Here's how the part is built. I have some questions about the finished solid (model axes, mm). Round coordinates to 2 decimals unless told otherwise and drop trailing zeros. Write each loop counter-clockwise with the first axis right and the second up, starting at its lowest first coordinate (ties: lowest second). Pieces come first, ordered by that corner, then holes. Notation, with made-up numbers: (21.25, -7) - (77.25, -7) arc R33 ccw to (77.25, 31) - close; hole circle Ø5 at (-37.75, 34). An arc over 180 degrees is marked (long way). Return JSON: item names as keys, results as strings. Group by question number.
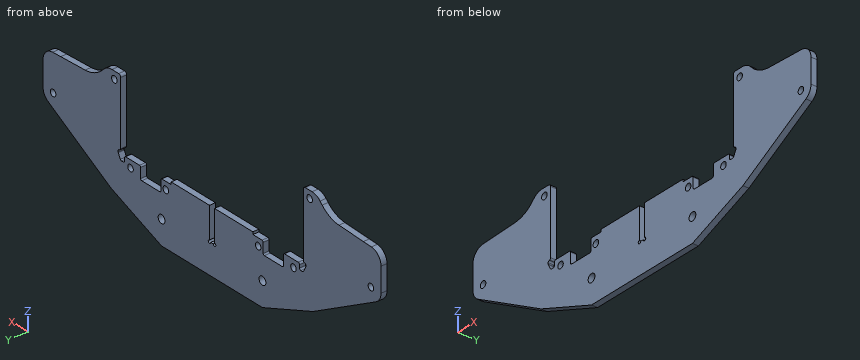
```python
from build123d import *

# Parameters (mm, degrees)
EXTRUDE_1_DEPTH      = 2
CUT_EXTRUDE_1_DEPTH  = 10
SKETCH_3_W           = 2
SKETCH_3_H           = 10
CUT_EXTRUDE_2_DEPTH  = 10
CUT_EXTRUDE_3_DEPTH  = 10
SKETCH_5_W           = 23
SKETCH_5_H           = 22.484633815
CUT_EXTRUDE_4_DEPTH  = 10
SKETCH_6_W           = 32.4
SKETCH_6_H           = 0.8
EXTRUDE_2_DEPTH      = 2
SKETCH_7_R           = 1.1
CUT_EXTRUDE_5_DEPTH  = 10
EXTRUDE_3_DEPTH      = 2
SKETCH_9_R           = 1.1
CUT_EXTRUDE_6_DEPTH  = 10
CHAMFER_2_SIZE       = 5
CHAMFER_2_SIZE_2     = 5.237723549
FILLET_2_R           = 10
FILLET_3_R           = 4.5
SKETCH_10_W          = 1.5
SKETCH_10_H          = 2
CUT_EXTRUDE_7_DEPTH  = 10
SKETCH_11_R          = 1.35
CUT_EXTRUDE_8_DEPTH  = 10
SKETCH_12_W          = 8
SKETCH_12_H          = 4.2
CUT_EXTRUDE_9_DEPTH  = 10
FILLET_5_R           = 0.45
CUT_EXTRUDE_10_DEPTH = 10
FILLET_6_R           = 0.5
FILLET_7_R           = 0.8
SKETCH_14_R          = 0.5
CUT_EXTRUDE_11_DEPTH = 10
SKETCH_15_W          = 2
SKETCH_15_H          = 0.8
CUT_EXTRUDE_12_DEPTH = 10
EXTRUDE_4_DEPTH      = 2
FILLET_8_R           = 4
SKETCH_17_R          = 1.1
CUT_EXTRUDE_13_DEPTH = 10


# Some blends are built 0.0001 mm under size
with BuildPart() as part:
    # 草图1 → 凸台-拉伸1 (new body)
    with BuildSketch(Plane(origin=(0, 0, 0), x_dir=(1, 0, 0), z_dir=(0, 1, 0))):
        Polygon((-20, 0), (20, 0), (60, -20), (60, -40), (0, -40), (-60, -40), (-60, -20), align=None)
    extrude(amount=EXTRUDE_1_DEPTH)

    # 草图2 → 切除-拉伸1 (cut)
    with BuildSketch(Plane(origin=(0, 2, 0), x_dir=(1, 0, 0), z_dir=(0, 1, 0))):
        Polygon((0, -20), (13.2, -20), (13.2, -40), (-13.2, -40), (-13.2, -20), align=None)
    extrude(amount=-CUT_EXTRUDE_1_DEPTH, mode=Mode.SUBTRACT)

    # 草图3 → 切除-拉伸2 (cut)
    with BuildSketch(Plane(origin=(0, 2, 0), x_dir=(1, 0, 0), z_dir=(0, 1, 0))):
        with Locations((0, -15)):
            Rectangle(SKETCH_3_W, SKETCH_3_H)
    extrude(amount=-CUT_EXTRUDE_2_DEPTH, mode=Mode.SUBTRACT)

    # 草图4 → 切除-拉伸3 (cut)
    with BuildSketch(Plane(origin=(0, 2, 0), x_dir=(1, 0, 0), z_dir=(0, 1, 0))):
        Polygon((-60, -40), (-60, -38), (-15, -40), align=None)
        Polygon((60, -40), (15, -40), (60, -38), align=None)
    extrude(amount=-CUT_EXTRUDE_3_DEPTH, mode=Mode.SUBTRACT)

    # 草图5 → 切除-拉伸4 (cut)
    with BuildSketch(Plane(origin=(0, 2, 0), x_dir=(1, 0, 0), z_dir=(0, 1, 0))):
        with Locations((24.7, -31.242316908)):
            Rectangle(SKETCH_5_W, SKETCH_5_H)
        with Locations((-24.7, -31.242316908)):
            Rectangle(SKETCH_5_W, SKETCH_5_H)
    extrude(amount=-CUT_EXTRUDE_4_DEPTH, mode=Mode.SUBTRACT)

    # 草图6 → 凸台-拉伸2 (add)
    with BuildSketch(Plane(origin=(0, 2, 0), x_dir=(1, 0, 0), z_dir=(0, 1, 0))):
        with Locations((0, -20.4)):
            Rectangle(SKETCH_6_W, SKETCH_6_H)
    extrude(amount=-EXTRUDE_2_DEPTH)

    # 草图7 → 切除-拉伸5 (cut)
    with BuildSketch(Plane(origin=(0, 2, 0), x_dir=(1, 0, 0), z_dir=(0, 1, 0))):
        with Locations(Location((32.3, -17.5, 0), (0, 0, 270))):
            Circle(SKETCH_7_R)
        with Locations(Location((18.3, -17.5, 0), (0, 0, 270))):
            Circle(SKETCH_7_R)
        with Locations(Location((-18.3, -17.5, 0), (0, 0, 90))):
            Circle(SKETCH_7_R)
        with Locations(Location((-32.3, -17.5, 0), (0, 0, 90))):
            Circle(SKETCH_7_R)
    extrude(amount=-CUT_EXTRUDE_5_DEPTH, mode=Mode.SUBTRACT)

    # 草图8 → 凸台-拉伸3 (add)
    with BuildSketch(Plane(origin=(0, 2, 0), x_dir=(1, 0, 0), z_dir=(0, 1, 0))):
        Polygon((-36.2, -43.5), (-36.2, -40), (-36.2, -35.5), (-41.2, -35.5), (-41.2, -43.5), align=None)
        Polygon((36.2, -40), (36.2, -35.5), (41.2, -35.5), (41.2, -43.5), (36.2, -43.5), align=None)
    extrude(amount=-EXTRUDE_3_DEPTH)

    # 草图9 → 切除-拉伸6 (cut)
    with BuildSketch(Plane(origin=(0, 2, 0), x_dir=(1, 0, 0), z_dir=(0, 1, 0))):
        with Locations(Location((38.7, -41, 0), (0, 0, 270))):
            Circle(SKETCH_9_R)
        with Locations(Location((-38.7, -41, 0), (0, 0, 90))):
            Circle(SKETCH_9_R)
    extrude(amount=-CUT_EXTRUDE_6_DEPTH, mode=Mode.SUBTRACT)

    # 倒角2
    # the kernel refuses this chamfer: 5.237723549, 5 mm, written as the material it adds along each edge
    with BuildSketch(Plane(origin=(-41.2, 2, 38.835555556), x_dir=(0.02876451379188079, 0, 0.9995862157644616), z_dir=(0, -1, 0))) as chamfer_2_piece_1_section:
        Polygon((CHAMFER_2_SIZE * 0.999586215764, CHAMFER_2_SIZE * 0.0287645137919), (-CHAMFER_2_SIZE_2 * 0.073118387756, CHAMFER_2_SIZE_2 * 0.997323268169), (0, 0), align=None)
    chamfer_2_piece_1 = extrude(amount=2, mode=Mode.PRIVATE)
    chamfer_2_piece_1 = split(chamfer_2_piece_1, bisect_by=Plane(origin=(-42.946846358, 1, 43.5), z_dir=(0, 0, -1)), keep=Keep.TOP, mode=Mode.PRIVATE)
    add(chamfer_2_piece_1)
    with BuildSketch(Plane(origin=(41.2, 2, 38.835555556), x_dir=(-0.028764513791882163, 0, 0.9995862157644615), z_dir=(0, -1, 0))) as chamfer_2_piece_2_section:
        Polygon((CHAMFER_2_SIZE * 0.999586215764, -CHAMFER_2_SIZE * 0.0287645137919), (-CHAMFER_2_SIZE_2 * 0.073118387756, -CHAMFER_2_SIZE_2 * 0.997323268169), (0, 0), align=None)
    chamfer_2_piece_2 = extrude(amount=2, mode=Mode.PRIVATE)
    chamfer_2_piece_2 = split(chamfer_2_piece_2, bisect_by=Plane(origin=(42.946846358, 1, 43.5), z_dir=(0, 0, -1)), keep=Keep.TOP, mode=Mode.PRIVATE)
    add(chamfer_2_piece_2)

    # 圆角2
    fillet_2_edges = [part.edges().sort_by_distance(p)[0] for p in [
        (-46.43255814, 1, 38.602997416),
        (46.43255814, 1, 38.602997416),
    ]]
    fillet(fillet_2_edges, radius=FILLET_2_R)

    # 圆角3
    fillet_3_edges = [part.edges().sort_by_distance(p)[0] for p in [
        (-41.535555556, 1, 43.5),
        (41.535555556, 1, 43.5),
    ]]
    fillet(fillet_3_edges, radius=FILLET_3_R)

    # 草图10 → 切除-拉伸7 (cut)
    with BuildSketch(Plane(origin=(0, 2, 0), x_dir=(1, 0, 0), z_dir=(0, 1, 0))):
        with Locations((35.45, -19)):
            Rectangle(SKETCH_10_W, SKETCH_10_H)
        with Locations((-35.45, -19)):
            Rectangle(SKETCH_10_W, SKETCH_10_H)
    extrude(amount=-CUT_EXTRUDE_7_DEPTH, mode=Mode.SUBTRACT)

    # 草图11 → 切除-拉伸8 (cut)
    with BuildSketch(Plane(origin=(0, 2, 0), x_dir=(1, 0, 0), z_dir=(0, 1, 0))):
        with Locations(Location((20, -8, 0), (0, 0, 270))):
            Circle(SKETCH_11_R)
        with Locations(Location((-20, -8, 0), (0, 0, 270))):
            Circle(SKETCH_11_R)
    extrude(amount=-CUT_EXTRUDE_8_DEPTH, mode=Mode.SUBTRACT)

    # 草图12 → 切除-拉伸9 (cut)
    with BuildSketch(Plane(origin=(0, 2, 0), x_dir=(1, 0, 0), z_dir=(0, 1, 0))):
        with Locations((-24.3, -17.9)):
            Rectangle(SKETCH_12_W, SKETCH_12_H)
        with Locations((24.3, -17.9)):
            Rectangle(SKETCH_12_W, SKETCH_12_H)
    extrude(amount=-CUT_EXTRUDE_9_DEPTH, mode=Mode.SUBTRACT)

    # 圆角5
    fillet_5_edges = [part.edges().sort_by_distance(p)[0] for p in [
        (20.3, 1, 20),
        (28.3, 1, 20),
        (-20.3, 1, 20),
        (-28.3, 1, 20),
        (-28.3, 1, 15.8),
        (-20.3, 1, 15.8),
        (28.3, 1, 15.8),
        (20.3, 1, 15.8),
    ]]
    fillet(fillet_5_edges, radius=FILLET_5_R)

    # 草图13 → 切除-拉伸10 (cut)
    with BuildSketch(Plane(origin=(0, 2, 0), x_dir=(1, 0, 0), z_dir=(0, 1, 0))):
        Polygon((-36.2, -18), (-36.2, -20), (-36.2, -21), (-37.2, -21), (-37.2, -20), align=None)
        Polygon((36.2, -21), (36.2, -20), (36.2, -18), (37.2, -20), (37.2, -21), align=None)
    extrude(amount=-CUT_EXTRUDE_10_DEPTH, mode=Mode.SUBTRACT)

    # 圆角6
    fillet_6_edges = [part.edges().sort_by_distance(p)[0] for p in [
        (34.7, 1, 20),
        (34.7, 1, 18),
        (36.2, 1, 18),
        (-34.7, 1, 18),
        (-34.7, 1, 20),
        (-36.2, 1, 18),
        (-37.2, 1, 20),
        (-36.2, 1, 21),
        (-37.2, 1, 21),
        (37.2, 1, 21),
        (36.2, 1, 21),
        (37.2, 1, 20),
    ]]
    fillet(fillet_6_edges, radius=FILLET_6_R - 0.0001)  # a hair under: the kernel refuses the full size

    # 圆角7
    fillet_7_edges = [part.edges().sort_by_distance(p)[0] for p in [
        (36.2, 1, 43.5),
        (-36.2, 1, 43.5),
    ]]
    fillet(fillet_7_edges, radius=FILLET_7_R)

    # 草图14 → 切除-拉伸11 (cut)
    with BuildSketch(Plane(origin=(0, 2, 0), x_dir=(1, 0, 0), z_dir=(0, 1, 0))):
        with Locations((-1, -10)):
            Circle(SKETCH_14_R)
        with Locations((1, -10)):
            Circle(SKETCH_14_R)
    extrude(amount=-CUT_EXTRUDE_11_DEPTH, mode=Mode.SUBTRACT)

    # 草图15 → 切除-拉伸12 (cut)
    with BuildSketch(Plane(origin=(0, 2, 0), x_dir=(1, 0, 0), z_dir=(0, 1, 0))):
        with Locations((0, -20.4)):
            Rectangle(SKETCH_15_W, SKETCH_15_H)
    extrude(amount=-CUT_EXTRUDE_12_DEPTH, mode=Mode.SUBTRACT)

    # 草图16 → 凸台-拉伸4 (add)
    with BuildSketch(Plane(origin=(0, 2, 0), x_dir=(1, 0, 0), z_dir=(0, 1, 0))):
        Polygon((-60, -20), (-60, -38), (-67, -37.688888889), (-67, -23.5), (-40, -8), (-20, 0), align=None)
        Polygon((40, -8), (67, -23.5), (67, -37.688888889), (60, -38), (60, -20), (20, 0), align=None)
    extrude(amount=-EXTRUDE_4_DEPTH)

    # 圆角8
    fillet_8_edges = [part.edges().sort_by_distance(p)[0] for p in [
        (-67, 1, 37.688888889),
        (-67, 1, 23.5),
        (67, 1, 23.5),
        (67, 1, 37.688888889),
    ]]
    fillet(fillet_8_edges, radius=FILLET_8_R)

    # 草图17 → 切除-拉伸13 (cut)
    with BuildSketch(Plane(origin=(0, 2, 0), x_dir=(1, 0, 0), z_dir=(0, 1, 0))):
        with Locations(Location((-63, -25.81596743, 0), (0, 0, 270))):
            Circle(SKETCH_17_R)
        with Locations(Location((63, -25.81596743, 0), (0, 0, 270))):
            Circle(SKETCH_17_R)
    extrude(amount=-CUT_EXTRUDE_13_DEPTH, mode=Mode.SUBTRACT)


solid = part.part
```
1) Imagine slicing it at B-B (y = 1.55). Give the number of separate pieces and of enclosed holes in the cut face, plus the area to 3 significant figures.
2) I need wall thicknesses on line 1 along X through (y, z) = (1.1, 8); line 2 along X through (y, z) = (0.25, 16); line 3 along X through (y, z) = (0.55, 41). Which ranges of each line are inside material? Lowest first, please.
3) Imagine slicing it at A-A (z = 13). Please give me the cut outline in (x, y), plus the area to 3 significant figures.
4) Will these pins go through, and if not, where does the flat tip stop? pin 1 Ø3 at (x, z) = (18.3, 17.5) entering from +Y; pin 2 Ø1 at (y, z) = (1.5, 17.5) entering from +X; pin 3 Ø1 at (x, y) = (18.5, 1) entering from +Z; pin 4 Ø0.6 at (x, y) = (35.5, 1) entering from +Z.
Results found:
{
 "1": {"separate pieces": "1", "enclosed holes": "10", "area": "2,750 mm²"},
 "2": {"line 1": "x = -40 to -21.35, -18.65 to 18.65, 21.35 to 40", "line 2": "x = -53.94 to -28.22, -20.38 to -1, 1 to 20.38, 28.22 to 53.94", "line 3": "x = -44.05 to -39.8, -37.6 to -36.2, 36.2 to 37.6, 39.8 to 44.05"},
 "3": {"outline": "(-48.71, 0) - (-1, 0) - (-1, 2) - (-48.71, 2) - close; (1, 0) - (48.71, 0) - (48.71, 2) - (1, 2) - close", "area": "191 mm²"},
 "4": {"pin 1": "stops at y = 2", "pin 2": "stops at x = 57.42", "pin 3": "stops at z = 20", "pin 4": "stops at z = 18"}
}
